Source: CAD feature listing. Evaluate the final solid. Frame: model axes, mm. Face numbers are marked on the shaded views. A direction names the side the tool comes from. Give positions to 0.01 mm unless a question says otherwise; leave off trailing zeros. Loops run counter-clockwise (first coordinate to the right, second up) from the corner with the lowest first, then second, coordinate; pieces in that order, holes last. Notation, with made-up numbers: (41.25, -4) - (56.25, -4) arc R3 ccw to (56.25, 1) - close; hole circle Ø5 at (17, -0.5). An arc over 180 degrees is marked (long way). Write each question's results on one line, items separated by ' | '. Start each with the question number.
(1) Reachability of the marked faces 5, 6 and 7 from +Z, -Z, +X, -X, +Y, -Y: full face, straight path, thin tool, end or side. Return the list, or none.
(2) Pull-direction query (Z, two-part tool) for the marked faces 1, 2, 3 and 4; classes: pulls with the +Z half, pulls with the -Z half, needs draft (parallel to the pull), parting line crosses it, or undercut.
(3) Cut plane C-C on x = -36. Return the cut outline in (y, z).
(4) Material intervals for line 1 along X through (y, z) = (38.5, 0) (3 decimals); line 2 along Z through (x, y) = (-2.5, 42.5) (1 decimal); line 3 along X through (y, z) = (18, -8.5), sorted ascending. Write a range as [from, to].
(5) Contact query for flat-ended pins moving along their axis: pin 1 (3 mm diameter, centred on x = -38.5, y = 8.5, fed in from -Z); pin 2 (10 mm diameter, centred on y = 43, z = 2.5, fed in from +X); pin 3 (5 mm diameter, centred on y = 6, z = 7.5, fed in from -X). Output: stop coordinate, or through.
(6) Cut plane B-B on z = 0. Return the cut outline in (x, y) (1 decimal).
(7) Cut plane A-A on y = 7. Return the cut outline in (x, z).
from build123d import *

# Parameters (mm, degrees)
SKETCH1_W                   = 25.4
SKETCH1_H                   = 25.4
BOSS_EXTRUDE1_DEPTH         = 21
SKETCH8_W                   = 2.902818519
SKETCH8_H                   = 9.580147983
BOSS_EXTRUDE4_DEPTH         = 25.4
SKETCH10_R                  = 12.7
BOSS_EXTRUDE5_DEPTH         = 29.7815
SKETCH12_R                  = 6.985
CUT_EXTRUDE2_DEPTH          = 22.9235
CHAMFER1_SIZE               = 2.54
SKETCH14_W                  = 12.7
SKETCH14_H                  = 25.4
BOSS_EXTRUDE6_DEPTH         = 15.24
CUT_EXTRUDE3_REACH          = 60.614
SKETCH18_W                  = 5.842
SKETCH18_H                  = 11.43
F_1_4_CLEARANCE_HOLE2_D     = 6.7564
F_1_4_CLEARANCE_HOLE2_DEPTH = 20.32
F_1_4_CLEARANCE_HOLE2_TIP   = 2.029827343
CHAMFER2_SIZE               = 10.16
SKETCH21_W                  = 5
SKETCH21_H                  = 21
BOSS_EXTRUDE7_DEPTH         = 42.5
SKETCH22_R                  = 2.64
CUT_EXTRUDE4_DEPTH          = 22


with BuildPart() as part:
    # Sketch1 → Boss-Extrude1 (new body)
    with BuildSketch(Plane(origin=(0, 0, 0), x_dir=(1, 0, 0), z_dir=(0, 1, 0))):
        Rectangle(SKETCH1_W, SKETCH1_H)
    extrude(amount=BOSS_EXTRUDE1_DEPTH)

    # Sketch8 → Boss-Extrude4 (add, through all)
    with BuildSketch(Plane.XY.offset(12.7)):
        with Locations((-1.45140926, 4.790073991)):
            Rectangle(SKETCH8_W, SKETCH8_H)
    extrude(amount=-BOSS_EXTRUDE4_DEPTH)

    # Sketch10 → Boss-Extrude5 (add)
    with BuildSketch(Plane(origin=(0, 21, 0), x_dir=(1, 0, 0), z_dir=(0, 1, 0))):
        with Locations(Location((0, 0, 0), (0, 0, 270))):
            Circle(SKETCH10_R)
    extrude(amount=BOSS_EXTRUDE5_DEPTH)

    # Sketch12 → Cut-Extrude2 (cut)
    with BuildSketch(Plane(origin=(0, 50.7815, 0), x_dir=(1, 0, 0), z_dir=(0, 1, 0))):
        with Locations(Location((0, 0, 0), (0, 0, 270))):
            Circle(SKETCH12_R)
    extrude(amount=-CUT_EXTRUDE2_DEPTH, mode=Mode.SUBTRACT)

    # Chamfer1
    chamfer1_edges = [part.edges().sort_by_distance(p)[0] for p in [
        (0, 50.7815, -12.7),
    ]]
    chamfer(chamfer1_edges, length=CHAMFER1_SIZE)

    # Sketch14 → Boss-Extrude6 (add)
    with BuildSketch(Plane.XY.offset(-6.985)):
        with Locations((0, 33.7)):
            Rectangle(SKETCH14_W, SKETCH14_H)
    extrude(amount=-BOSS_EXTRUDE6_DEPTH)

    # Sketch18 → Cut-Extrude3 (cut, up to next)
    with BuildSketch(Plane(origin=(6.35, 0, 0), x_dir=(0, 0, -1), z_dir=(1, 0, 0)), mode=Mode.PRIVATE) as cut_extrude3_sk1:
        with Locations((16.149395763, 36.875)):
            Rectangle(SKETCH18_W, SKETCH18_H)
    cut_extrude3_tool1 = extrude(cut_extrude3_sk1.sketch, amount=-CUT_EXTRUDE3_REACH, mode=Mode.PRIVATE) & part.part
    add(cut_extrude3_tool1.solids().sort_by_distance((6.35, 36.875, -16.149396))[0], mode=Mode.SUBTRACT)

    # 1/4 Clearance Hole2
    with Locations(Plane(origin=(0, 0, -22.225), x_dir=(-1, 0, 0), z_dir=(0, 0, -1))):
        with Locations((0, 36.875)):
            Hole(F_1_4_CLEARANCE_HOLE2_D / 2, depth=F_1_4_CLEARANCE_HOLE2_DEPTH)
            with Locations((0, 0, -(F_1_4_CLEARANCE_HOLE2_DEPTH + F_1_4_CLEARANCE_HOLE2_TIP / 2))):  # 118° drill point
                Cone(0, F_1_4_CLEARANCE_HOLE2_D / 2, F_1_4_CLEARANCE_HOLE2_TIP, mode=Mode.SUBTRACT)

    # Chamfer2
    # the kernel refuses this chamfer: 10.16 mm, written as the material it takes off along each edge
    with BuildSketch(Plane(origin=(32.478299158, 21, -22.225), x_dir=(0, 0.9996219169112968, -0.027495876610586268), z_dir=(-1, 0, 0))) as chamfer2_piece_1_section:
        Polygon((CHAMFER2_SIZE * 0.999621916911, -CHAMFER2_SIZE * 0.0274958766106), (-CHAMFER2_SIZE * 0.0274958766106, -CHAMFER2_SIZE * 0.999621916911), (0, 0), align=None)
    chamfer2_piece_1 = extrude(amount=64.956598315, mode=Mode.PRIVATE)
    chamfer2_piece_1 = split(chamfer2_piece_1, bisect_by=Plane(origin=(0, 24.386079735, -12.7), z_dir=(0, 0, -1)), keep=Keep.TOP, mode=Mode.PRIVATE)
    add(chamfer2_piece_1, mode=Mode.SUBTRACT)

    # Sketch21 → Boss-Extrude7 (add)
    with BuildSketch(Plane(origin=(12.7, 0, 0), x_dir=(0, 0, -1), z_dir=(1, 0, 0))):
        with Locations((-0.183594793, 10.5)):
            Rectangle(SKETCH21_W, SKETCH21_H)
    boss_extrude7 = extrude(amount=BOSS_EXTRUDE7_DEPTH)

    # Sketch22 → Cut-Extrude4 (cut)
    with BuildSketch(Plane(origin=(0, 0, 0), x_dir=(-1, 0, 0), z_dir=(0, -1, 0))):
        with Locations(Location((0, 0, 0), (0, 0, 90))):
            Circle(SKETCH22_R)
    extrude(amount=-CUT_EXTRUDE4_DEPTH, mode=Mode.SUBTRACT)

    # Mirror1: Boss-Extrude7 across plane
    add(boss_extrude7.mirror(Plane(origin=(0, 0, 0), x_dir=(0, 0, 1), z_dir=(1, 0, 0))))


solid = part.part
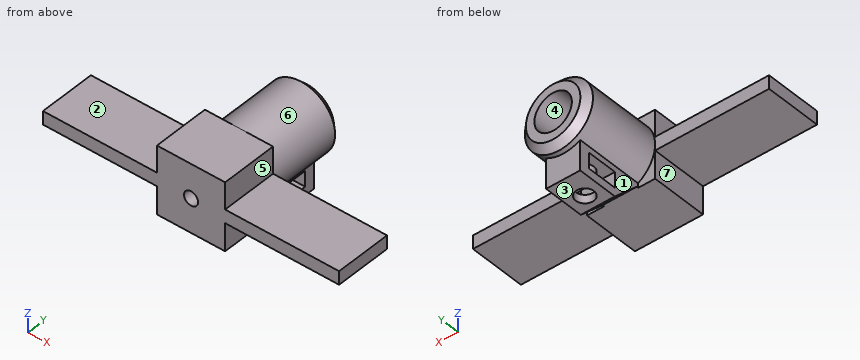
Ans:
1) face 5: +Z, +X, +Y, -Y | face 6: +Y | face 7: -Z, -X, +Y, -Y
2) face 1: needs draft | face 2: pulls with the +Z half | face 3: pulls with the -Z half | face 4: undercut
3) outline: (0, -2.32) - (21, -2.32) - (21, 2.68) - (0, 2.68) - close
4) line 1: [-12.7, -6.985], [6.985, 12.7] | line 2: [-22.2, -19.1], [-13.2, -6.5], [6.5, 12.5] | line 3: [-12.7, 12.7]
5) pin 1: z = -2.32 | pin 2: x = 12.7 | pin 3: x = -12.7
6) outline: (-55.2, 0) - (-2.6, 0) - (-2.6, 22) - (2.6, 22) - (2.6, 0) - (55.2, 0) - (55.2, 21) - (12.7, 21) - (12.7, 48.2) - (10.2, 50.8) - (7, 50.8) - (7, 27.9) - (-7, 27.9) - (-7, 50.8) - (-10.2, 50.8) - (-12.7, 48.2) - (-12.7, 21) - (-55.2, 21) - close
7) outline: (-55.2, -2.32) - (-12.7, -2.32) - (-12.7, -12.7) - (12.7, -12.7) - (12.7, -2.32) - (55.2, -2.32) - (55.2, 2.68) - (12.7, 2.68) - (12.7, 12.7) - (-12.7, 12.7) - (-12.7, 2.68) - (-55.2, 2.68) - close; hole circle Ø5.28 at (0, 0)
